Work out the finished part from the listing and answer in its coordinate system (mm). Face numbers are marked on the shaded views. Give positions to 0.01 mm unless a question says otherwise; leave off trailing zeros. Write each loop counter-clockwise with the first axis right and the second up, starting at its lowest first coordinate (ties: lowest second). Pieces come first, ordered by that corner, then holes. Notation, with made-up numbers: (78, 26) -> (108, 26) arc R17 ccw to (108, 46) -> close; hole circle Ø9 at (38, 21.5). An arc over 180 degrees is marked (long way). Use a Markdown table: item, result. Add a question column.
Q1. Section C-C, the plane y = 11 is taken. Give the vertices of the cut face in (x, z), plus the area to 3 significant figures.
Q2. Section B-B, the plane x = 10 is taken. Give the vertices of the cut face in (y, z) (3 decimals), plus the area to 3 significant figures.
Q3. Each of these flat-tipped pins is pushed along its axis until it touches: pin 1 Ø10 at (x, z) = (6, -3.5) entering from +Y; pin 2 Ø3 at (y, z) = (15, -15.5) entering from -X; pin 3 Ø3 at (y, z) = (13, 13) entering from -X; pin 4 Ø2.5 at (x, z) = (10, 15) entering from -Y. Where does it stop, or does it pass through?
Q4. Section A-A, the plane z = -15 is taken. Give the vertices of the cut face in (x, y) (3 decimals).
Q5. Consider line 1 (X direction, y = 2.05, z = 15) (3 decimals); line 2 (Z direction, x = 33.5, y = 8.75); line 3 (Z direction, x = 26, y = 17.25). Determine where each line is inside the solid, lowest interval first.
Q6. Section D-D, the plane x = 15.5 is taken. Give the vertices of the cut face in (y, z), plus the area to 3 significant figures.
Q7. For a pull along Z with two mould halves and no side action, classify the marked faces 1, 2 and 3 as pulls with the +Z half, pulls with the -Z half, needs draft (parallel to the pull), parting line crosses it, or undercut.
from build123d import *

# Parameters (mm, degrees)
SKETCH_1_W          = 50
SKETCH_1_H          = 30.1
EXTRUDE_1_DEPTH     = 70
CUT_EXTRUDE_2_DEPTH = 70
DRAFT_4_ANGLE       = 1.591
SKETCH_4_W          = 61.588766385
SKETCH_4_H          = 50
CUT_EXTRUDE_3_DEPTH = 93.871109174
SHELL_2_T           = -3
SKETCH_5_R          = 2.125
CUT_EXTRUDE_4_DEPTH = 64.356474986


with BuildPart() as part:
    # 草圖1 → 填料-伸長1 (new body)
    with BuildSketch(Plane(origin=(0, 0, 0), x_dir=(1, 0, 0), z_dir=(0, 1, 0))):
        with Locations((25, 15.05)):
            Rectangle(SKETCH_1_W, SKETCH_1_H)
    extrude_1 = extrude(amount=EXTRUDE_1_DEPTH)

    # 草圖3 → 除料-伸長2 (cut)
    with BuildSketch(Plane(origin=(0, 70, 0), x_dir=(1, 0, 0), z_dir=(0, 1, 0))):
        with BuildLine():
            Line((20, 30.1), (50, 30.1))
            Line((50, 30.1), (50, 0.1))
            ThreePointArc((50, 0.1), (28.786796564, 8.886796564), (20, 30.1))
        make_face()
    cut_extrude_2 = extrude(amount=-CUT_EXTRUDE_2_DEPTH, mode=Mode.SUBTRACT)

    # 鏡射1: 填料-伸長1, 除料-伸長2 across plane
    add(extrude_1.mirror(Plane.XY))
    add(cut_extrude_2.mirror(Plane.XY), mode=Mode.SUBTRACT)

    # 拔模4
    draft_4_faces = [part.faces().sort_by_distance(p)[0] for p in [
        (50, 35, 0),
        (10, 35, 30.1),
        (28.786796564, 35, 8.886796564),
    ]]
    draft(draft_4_faces, Plane.ZX.offset(70), DRAFT_4_ANGLE)

    # 草圖4 → 除料-伸長3 (cut, through all)
    with BuildSketch(Plane.ZY):
        with Locations((0.694383193, 45)):
            Rectangle(SKETCH_4_W, SKETCH_4_H)
    extrude(amount=-CUT_EXTRUDE_3_DEPTH, mode=Mode.SUBTRACT)

    # 薄殼2
    shell_2_openings = [part.faces().sort_by_distance(p)[0] for p in [
        (10.858708279, 9.954778556, 31.767775702),
        (14.773415442, 20, 0.973960422),
        (10, 10, -30.1),
        (0, 9.985034809, 0.833467662),
    ]]
    offset(amount=SHELL_2_T, openings=shell_2_openings, kind=Kind.INTERSECTION)

    # 草圖5 → 除料-伸長4 (cut, through all)
    with BuildSketch(Plane(origin=(0, 3, 0), x_dir=(1, 0, 0), z_dir=(0, 1, 0))):
        with Locations(Location((10, 15, 0), (0, 0, 270))):
            Circle(SKETCH_5_R)
        with Locations(Location((10, -15, 0), (0, 0, 90))):
            Circle(SKETCH_5_R)
    extrude(amount=-CUT_EXTRUDE_4_DEPTH, mode=Mode.SUBTRACT)


solid = part.part
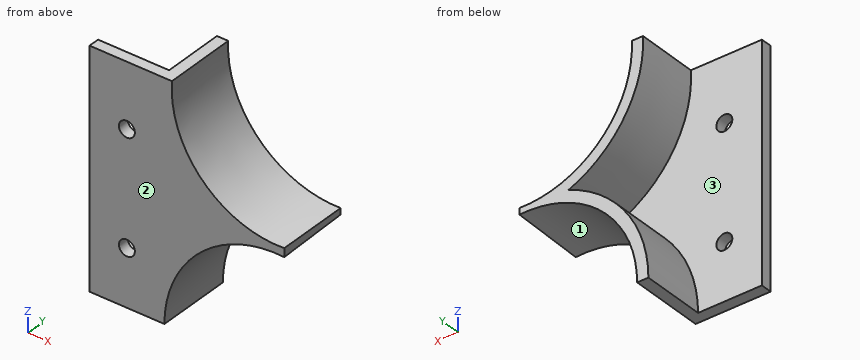
Result set:
| question | item | result |
|---|---|---|
| 1 | outline | (17, -30.1) -> (20, -30.1) arc R30 cw to (51.64, -0.14) -> (51.64, 1.79) arc R28.36 cw to (21.69, 31.74) -> (18.68, 31.74) arc R31.36 ccw to (38.62, 0.88) arc R33 ccw to start |
| 1 | area | 265 mm2 |
| 2 | outline | (0, -30.1) -> (3, -30.1) -> (3, -17.125) -> (0, -17.125) -> close; (0, -12.875) -> (3, -12.875) -> (3, 12.875) -> (0, 12.875) -> close; (0, 17.125) -> (3, 17.125) -> (3, 31.961) -> (0, 32.044) -> close |
| 2 | area | 161 mm2 |
| 3 | pin 1 | stops at y = 3 |
| 3 | pin 2 | stops at x = 19.71 |
| 3 | pin 3 | stops at x = 22.73 |
| 3 | pin 4 | passes through |
| 4 | outline | (0, 0) -> (7.875, 0) -> (7.875, 3) -> (0, 3) -> close; (12.125, 0) -> (24.077, 0) -> (24.077, 20) -> (20.657, 20) -> (20.657, 3) -> (12.125, 3) -> close |
| 5 | line 1 | x = 0 to 7.875, 12.125 to 26.287 |
| 5 | line 2 | z = -5.05 to -1.52, 3.5 to 7.11 |
| 5 | line 3 | z = -12.1 to -7.45, 9.64 to 14.67 |
| 6 | outline | (0, -30.1) -> (3, -30.1) -> (3, 31.96) -> (0, 32.04) -> close |
| 6 | area | 186 mm2 |
| 7 | face 1 | pulls with the -Z half |
| 7 | face 2 | needs draft |
| 7 | face 3 | undercut |
